```python
from build123d import *

# Parameters (mm, degrees)
SALIENTE_EXTRUIR1_DEPTH = 3.5
CROQUIS2_R              = 13.5
SALIENTE_EXTRUIR2_DEPTH = 5
CROQUIS4_R              = 18.5
CROQUIS5_R              = 13.5
CROQUIS6_R              = 18.5
SALIENTE_EXTRUIR3_DEPTH = 10
CROQUIS7_W              = 10
CROQUIS7_H              = 14
SALIENTE_EXTRUIR4_DEPTH = 9.335
SALIENTE_EXTRUIR5_DEPTH = 7
SALIENTE_EXTRUIR6_START = -15
SALIENTE_EXTRUIR6_DEPTH = 15
SALIENTE_EXTRUIR7_DEPTH = 8
CROQUIS11_R             = 1.5
CORTAR_EXTRUIR1_DEPTH   = 104.624142837


# Read off the part's stored shape, not the designer's step: Saliente-Extruir6
with BuildPart() as part:
    # Croquis1 → Saliente-Extruir1 (new body)
    with BuildSketch(Plane(origin=(0, 0, 0), x_dir=(1, 0, 0), z_dir=(0, 1, 0))):
        with BuildLine():
            Line((13.865110625, -13.711626722), (60.412611283, -13.711626722))
            Line((60.412611283, -13.711626722), (60.412611283, 16.288373278))
            Line((60.412611283, 16.288373278), (10.720955925, 16.288373278))
            ThreePointArc((10.720955925, 16.288373278), (14.366212875, 13.1856713), (17.145731884, 9.288373278))
            Line((17.145731884, 9.288373278), (53.412611283, 9.288373278))
            Line((53.412611283, 9.288373278), (53.412611283, -6.711626722))
            Line((53.412611283, -6.711626722), (18.308579048, -6.711626722))
            ThreePointArc((18.308579048, -6.711626722), (16.463188536, -10.450522629), (13.865110625, -13.711626722))
        make_face()
        with BuildLine():
            Line((-18.308579048, -6.711626722), (18.308579048, -6.711626722))
            ThreePointArc((18.308579048, -6.711626722), (19.199834523, -3.408277319), (19.5, 0))
            ThreePointArc((19.5, 0), (18.902271976, 4.791045202), (17.145731884, 9.288373278))
            Line((17.145731884, 9.288373278), (-17.145731884, 9.288373278))
            ThreePointArc((-17.145731884, 9.288373278), (-19.448702808, 1.413491806), (-18.308579048, -6.711626722))
        make_face()
        with BuildLine():
            ThreePointArc((17.145731884, 9.288373278), (14.366212875, 13.1856713), (10.720955925, 16.288373278))
            Line((10.720955925, 16.288373278), (-10.720955925, 16.288373278))
            ThreePointArc((-10.720955925, 16.288373278), (-14.366212875, 13.1856713), (-17.145731884, 9.288373278))
            Line((-17.145731884, 9.288373278), (17.145731884, 9.288373278))
        make_face()
        with BuildLine():
            Line((-13.865110625, -13.711626722), (13.865110625, -13.711626722))
            ThreePointArc((13.865110625, -13.711626722), (16.463188536, -10.450522629), (18.308579048, -6.711626722))
            Line((18.308579048, -6.711626722), (-18.308579048, -6.711626722))
            ThreePointArc((-18.308579048, -6.711626722), (-16.463188536, -10.450522629), (-13.865110625, -13.711626722))
        make_face()
        with BuildLine():
            ThreePointArc((-13.865110625, -13.711626722), (0, -19.5), (13.865110625, -13.711626722))
            Line((13.865110625, -13.711626722), (-13.865110625, -13.711626722))
        make_face()
        with BuildLine():
            Line((-10.720955925, 16.288373278), (10.720955925, 16.288373278))
            ThreePointArc((10.720955925, 16.288373278), (0, 19.5), (-10.720955925, 16.288373278))
        make_face()
    extrude(amount=SALIENTE_EXTRUIR1_DEPTH)

    # Croquis2 → Saliente-Extruir2 (add)
    with BuildSketch(Plane(origin=(0, 3.5, 0), x_dir=(1, 0, 0), z_dir=(0, 1, 0))):
        with Locations(Location((0, 0, 0), (0, 0, 270))):
            Circle(CROQUIS2_R)
    extrude(amount=SALIENTE_EXTRUIR2_DEPTH)

    # Croquis4 → Recubrir2 section 0
    with BuildSketch(Plane(origin=(0, 18.5, 0), x_dir=(1, 0, 0), z_dir=(0, 1, 0))):
        Circle(CROQUIS4_R)
    # Croquis5 → Recubrir2 section 1
    with BuildSketch(Plane(origin=(0, 8.5, 0), x_dir=(1, 0, 0), z_dir=(0, 1, 0))):
        Circle(CROQUIS5_R)
    loft()

    # Croquis6 → Saliente-Extruir3 (add)
    with BuildSketch(Plane(origin=(0, 18.5, 0), x_dir=(1, 0, 0), z_dir=(0, 1, 0))):
        with Locations(Location((0, 0, 0), (0, 0, 270))):
            Circle(CROQUIS6_R)
    extrude(amount=SALIENTE_EXTRUIR3_DEPTH)

    # Croquis7 → Saliente-Extruir4 (add)
    with BuildSketch(Plane(origin=(0, 28.5, 0), x_dir=(1, 0, 0), z_dir=(0, 1, 0))):
        with Locations((-8.995895444, 0)):
            Rectangle(CROQUIS7_W, CROQUIS7_H)
    extrude(amount=SALIENTE_EXTRUIR4_DEPTH)

    # Croquis8 → Saliente-Extruir5 (add, symmetric)
    with BuildSketch(Plane.XY):
        Polygon((-13.995895444, 37.835), (-13.995895444, 43.365), (1.004104556, 43.365), (-3.995895444, 37.835), align=None)
    extrude(amount=SALIENTE_EXTRUIR5_DEPTH, both=True)

    # Saliente-Extruir6 outline → Saliente-Extruir6 (add)
    with BuildSketch(Plane.ZY.offset(13.995895444).offset(SALIENTE_EXTRUIR6_START)):
        with BuildLine():
            Line((7, 43.365), (7, 43.363083448))
            ThreePointArc((7, 43.363083448), (-0.197524964, 69.433648419), (-7, 43.257226645))
            Line((-7, 43.257226645), (-7, 43.365))
            Line((-7, 43.365), (7, 43.365))
        make_face()
    extrude(amount=SALIENTE_EXTRUIR6_DEPTH)

    # Croquis10 → Saliente-Extruir7 (add, symmetric)
    with BuildSketch(Plane.XY):
        Polygon((58.412611283, 3.5), (54.412611283, 3.5), (54.412611283, 12.42), (41.356500297, 19.957949192), (42.831821975, 22.513281297), (58.420279243, 13.513281297), (58.412611283, 13.5), align=None)
    extrude(amount=SALIENTE_EXTRUIR7_DEPTH, both=True)

    # Croquis11 → Cortar-Extruir1 (cut, through all)
    with BuildSketch(Plane.ZY.offset(13.995895444)):
        with Locations((-1.591671186, 59.434048604)):
            Circle(CROQUIS11_R)
        with Locations((1.408328814, 51.434048604)):
            Circle(CROQUIS11_R)
    extrude(amount=-CORTAR_EXTRUIR1_DEPTH, mode=Mode.SUBTRACT)


solid = part.part
```
Can you work these out from the model? Positions are in its coordinate system, mm. A direction names the side the tool comes from. Coordinates: 2 decimals unless noted, no trailing zeros. Write each loop counter-clockwise with the first axis right and the second up, starting at its lowest first coordinate (ties: lowest second). Pieces come first, ordered by that corner, then holes. Notation, with made-up numbers: (65.5, 58) - (84.5, 58) arc R26 ccw to (84.5, 78) - close; hole circle Ø6 at (15.5, 13). An arc over 180 degrees is marked (long way). Return JSON: item names as keys, results as strings.
Q1. Thinking about a two-plate mould opening in Y: for faces 1 (the flat face through (50.517, 18.076, 0.112)), 2 (the flat face through (1.004, 57, 0)), 3 (the flat face through (-3.996, 33, 0)), which applies, +Y half, -Y half, draft (parallel to the pull), parting line (faces both ways), or undercut?
Computed values:
{"face 1": "+Y half", "face 2": "draft", "face 3": "undercut"}
Q2. Please list where these lines run through material, in increasing order: L1, parallel to X at y = 44, z = 3; L2, parallel to Z at x = -7, y = 25; L3, parallel to Y at x = 31.5, z = -16. Write a range as from..to.
Computed values:
{"L1": "x = -14..1", "L2": "z = -17.12..17.12", "L3": "y = 0..3.5"}
Q3. On a 3-axis mill with a long thin cutter (end or side, diameter ignored), from which of +Z, -Z, +X, -X, +Y, -Y can I reach the whole of each face in a straight line? I mean faces 4 (the flat face through (54.413, 8, 0)), 5 (the flat face through (52, 14, 8)), 6 (the cylindrical face through (-13.18, 5.96, -2.93)), 7 (the flat face through (42.084, 21.218, 0.112)). Say none if no direction works.
Computed values:
{"face 4": "+Z, -Z", "face 5": "+Z, +X, +Y", "face 6": "none", "face 7": "+Z, -Z, +Y"}
Q4. I'm going to push flat-ended pins straight in: pin 1 Ø8 at (x, y) = (-9.5, 35) entering from +Z; pin 2 Ø1.5 at (x, z) = (5.5, -12) entering from -Y; pin 3 Ø8 at (x, z) = (7.5, 8.5) entering from +Y; pin 4 Ø8 at (x, z) = (-3.5, -15.5) entering from +Y. Where does each tip first touch, or does it pass through?
Computed values:
{"pin 1": "stops at z = 7", "pin 2": "stops at y = 0", "pin 3": "stops at y = 28.5", "pin 4": "stops at y = 63.55"}
Q5. If we section it at A-A (x = 23): Please give me the cut outline in (y, z), then the cut area to 3 significant figures.
Computed values:
{"outline": "(0, -16.29) - (3.5, -16.29) - (3.5, -9.29) - (0, -9.29) - close; (0, 6.71) - (3.5, 6.71) - (3.5, 13.71) - (0, 13.71) - close", "area": "49.0 mm2"}
Q6. If we section it at C-C (y = 15.5): Please give me the cut outline in (x, z).
Computed values:
{"outline": "circle Ø34 at (0, 0); (49.08, -8) - (54.98, -8) - (54.98, 8) - (49.08, 8) - close"}
Q7. If we section it at B-B (x = 0): Please give me the cut outline in (y, z), then the cut area to 3 significant figures.
Computed values:
{"outline": "(0, -19.5) - (3.5, -19.5) - (3.5, -13.5) - (8.5, -13.5) - (18.5, -18.5) - (28.5, -18.5) - (28.5, 18.5) - (18.5, 18.5) - (8.5, 13.5) - (3.5, 13.5) - (3.5, 19.5) - (0, 19.5) - close; (42.25, -7) - (43.26, -7) arc R14 ccw (long way) to (43.36, 7) - (42.25, 7) - close; hole circle Ø3 at (51.43, 1.41); hole circle Ø3 at (59.43, -1.59)", "area": "1,560 mm2"}
Q8. If we section it at D-D (x = 46): Please give me the cut outline in (y, z).
Computed values:
{"outline": "(0, -16.29) - (3.5, -16.29) - (3.5, -9.29) - (0, -9.29) - close; (0, 6.71) - (3.5, 6.71) - (3.5, 13.71) - (0, 13.71) - close; (17.28, -8) - (20.68, -8) - (20.68, 8) - (17.28, 8) - close"}
